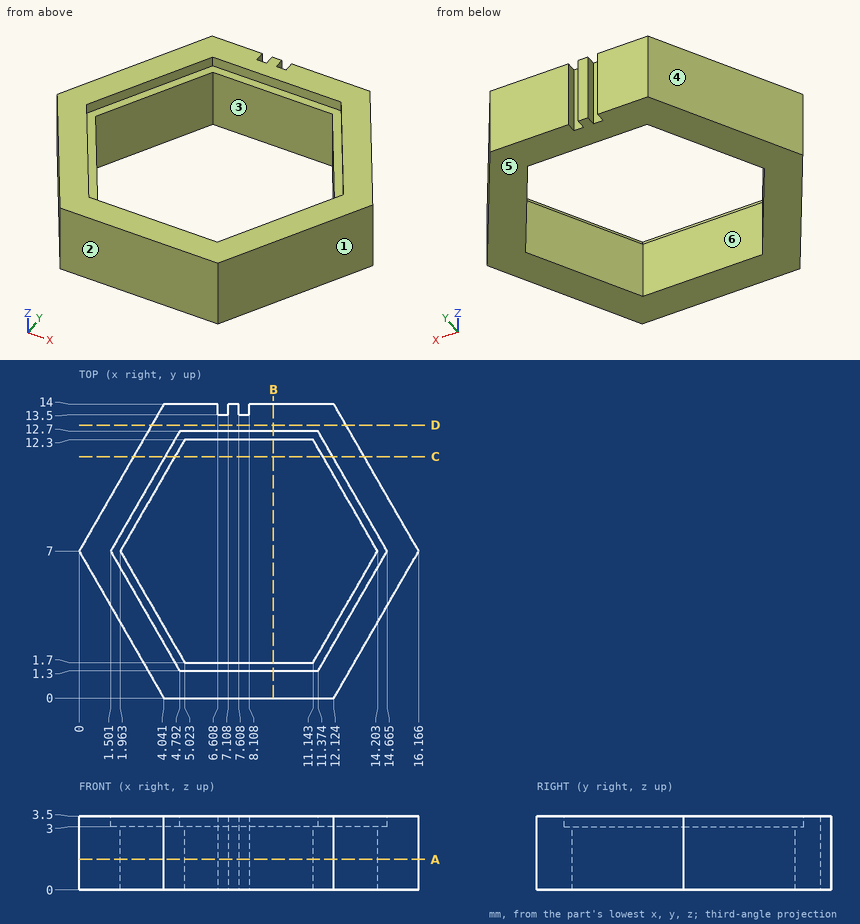
Study the drawing (mm; zero at the part's minimum x, y, z) and answer. A direction names the side the tool comes from. Give positions to 0.01 mm unless a question says otherwise; leave off trailing zeros. Write each loop counter-clockwise with the first axis right and the second up, starting at its lowest first coordinate (ties: lowest second). Pieces come first, ordered by that corner, then holes. Notation, with made-up numbers: M 53,-28 L 67,-28 A10 cw 67,-20 Z; hole C 56.25,-35 d9. An arc over 180 degrees is marked long. Put each result on its own line as item: value. Start each with the question number.
1. For a pull along X with two mould halves and no side action, classify the marked faces 1, 2, 3 and 4 as released by +X, released by -X, zero draft, split by the parting line, or undercut.
2. The part is cut by section B-B, the plane x = 9.25. Give the vertices of the cut face in (y, z), and give its area (3 significant figures).
3. The part is cut by section A-A, the plane z = 1.45. Give the vertices of the cut face in (x, y) (1 decimal).
4. The part is cut by section C-C, the plane y = 11.5. Give the vertices of the cut face in (x, z) (1 decimal).
5. Which of the six approach directions +Z, -Z, +X, -X, +Y, -Y give full straight-line access (tool end or side, diameter ignored) to the marked faces 5 and 6?
6. Each of these flat-tipped pins is pushed along its axis until it touches: pin 1 Ø1 at (x, y) = (9.5, 4) entering from +Z; pin 2 Ø0.6 at (y, z) = (13.5, 1) entering from -X; pin 3 Ø0.6 at (y, z) = (14, 1) entering from -X. Where does it stop, or does it pass through?
7. The part is cut by section D-D, the plane y = 13. Give the vertices of the cut face in (x, z) (1 decimal).
8. Consider line 1 along Y through (x, z) = (7.5, 2.8); line 2 along Y through (x, z) = (3, 0.7) (1 decimal); line 3 along X through (y, z) = (6.25, 1.9) (1 decimal). Determine where each line is inside the solid, lowest interval first.
Final values:
1. face 1: released by +X
1. face 2: zero draft
1. face 3: undercut
1. face 4: released by -X
2. outline: M 0,0 L 1.7,0 L 1.7,3 L 1.3,3 L 1.3,3.5 L 0,3.5 Z; M 12.3,0 L 14,0 L 14,3.5 L 12.7,3.5 L 12.7,3 L 12.3,3 Z
2. area: 11.5 mm²
3. outline: M 0,7 L 4,0 L 12.1,0 L 16.2,7 L 12.1,14 L 8.1,14 L 8.1,13.5 L 7.6,13.5 L 7.6,14 L 7.1,14 L 7.1,13.5 L 6.6,13.5 L 6.6,14 L 4,14 Z; hole M 2,7 L 5,1.7 L 11.1,1.7 L 14.2,7 L 11.1,12.3 L 5,12.3 Z
4. outline: M 2.6,0 L 4.6,0 L 4.6,3 L 4.1,3 L 4.1,3.5 L 2.6,3.5 Z; M 11.6,0 L 13.6,0 L 13.6,3.5 L 12.1,3.5 L 12.1,3 L 11.6,3 Z
5. face 5: -Z, +X, -X, +Y, -Y
5. face 6: +Z, -Z
6. pin 1: passes through
6. pin 2: stops at x = 3.58
6. pin 3: stops at x = 3.87
7. outline: M 3.5,0 L 12.7,0 L 12.7,3.5 L 3.5,3.5 Z
8. line 1: y = 0 to 1.7, 12.3 to 14
8. line 2: y = 1.8 to 5.2, 8.8 to 12.2
8. line 3: x = 0.4 to 2.4, 13.8 to 15.7
